```python
from build123d import *

# Parameters (mm, degrees)
SKETCH_1_R      = 10
EXTRUDE_1_DEPTH = 20
SKETCH_3_R      = 9
EXTRUDE_3_DEPTH = 20


with BuildPart() as part:
    # 草圖1 → 填料-伸長1 (new body)
    with BuildSketch(Plane(origin=(0, 0, 0), x_dir=(1, 0, 0), z_dir=(0, 1, 0))):
        with BuildLine():
            Line((0, 0), (150, 0))
            Line((150, 0), (150, -48.937372985))
            ThreePointArc((150, -48.937372985), (142.306045532, -66.979013377), (123.959936956, -73.915728993))
            Line((123.959936956, -73.915728993), (14.009507708, -39.398116187))
            ThreePointArc((14.009507708, -39.398116187), (3.878432988, -32.15252135), (0, -20.316344726))
            Line((0, -20.316344726), (0, 0))
        make_face()
        with Locations(Location((20, -19.398116187, 0), (0, 0, 270))):
            Circle(SKETCH_1_R, mode=Mode.SUBTRACT)
        with Locations(Location((125, -48.915728993, 0), (0, 0, 270))):
            Circle(SKETCH_1_R, mode=Mode.SUBTRACT)
    extrude(amount=EXTRUDE_1_DEPTH)

    # 草圖3 → 填料-伸長3 (add)
    with BuildSketch(Plane(origin=(0, 0, 0), x_dir=(-1, 0, 0), z_dir=(0, 0, -1))):
        with BuildLine():
            Line((-150, 20), (-150, 50.956093838))
            ThreePointArc((-150, 50.956093838), (-147.247819565, 58.603173888), (-140.253694451, 62.742563256))
            Line((-140.253694451, 62.742563256), (-79.695196774, 74.321972269))
            ThreePointArc((-79.695196774, 74.321972269), (-59.068583229, 69.033118411), (-50, 49.76682765))
            Line((-50, 49.76682765), (-50, 20))
            Line((-50, 20), (-150, 20))
        make_face()
        with Locations((-75, 49.76682765)):
            Circle(SKETCH_3_R, mode=Mode.SUBTRACT)
    extrude(amount=-EXTRUDE_3_DEPTH)


solid = part.part
```
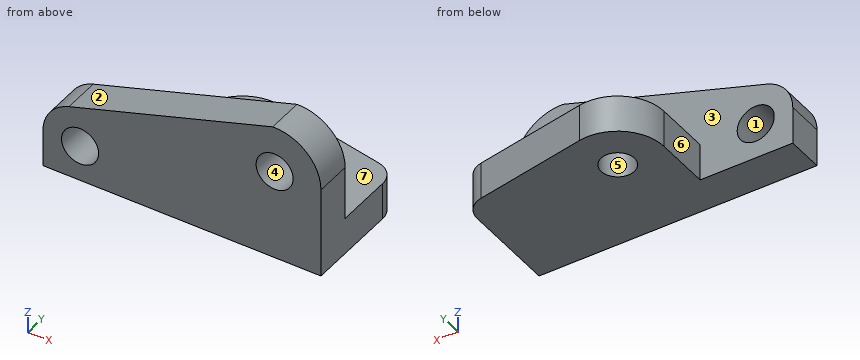
The model under review builds one solid part; all positions refer to its coordinate system, in mm. Face numbers are marked on the shaded views. A direction names the side the tool comes from. Round coordinates to 2 decimals unless told otherwise and drop trailing zeros. Write each loop counter-clockwise with the first axis right and the second up, starting at its lowest first coordinate (ties: lowest second). Pieces come first, ordered by that corner, then holes. Notation, with made-up numbers: M -25.5,-16.75 L 18.5,-16.75 A30 ccw 18.5,16.25 Z; hole C -3,57.5 d7. An arc over 180 degrees is marked long. Use CSV: the item, a comma, the result in double quotes. Start each with the question number.
(1) We need section C-C, the plane z = 54. State the section outline as (x, y) points, then the cut area to 3 significant figures.
(2) Clearance check with flat-ended pins moving along their axes: P1, Ø5, axis at x = 110.5, y = 51.5, coming from the +Z side; P2, Ø8, axis at y = 54, z = 13.5, coming from the +X side; P3, Ø1, axis at x = 117, y = 15.5, coming from the +Z side; P4, Ø6, axis at x = 64.5, z = 13, coming from the +Y side. State where each tip first meets the part, or that it passes through.
(3) Tool access review of the marked faces 5, 6 and 7: name each direction out of +Z, -Z, +X, -X, +Y, -Y from which nothing blocks a thin tool from reaching the whole face with its end or side.
(4) We need section A-A, the plane y = 18. State the section outline as (x, z) points.
(5) We need section D-D, the plane z = 5. State the section outline as (x, y) points, then the cut area to 3 significant figures.
(6) The part is to be moulded in two halves that separate along Z. For the marked faces 1, 2, 3 and 4, say which applies: +Z half, -Z half, draft (parallel to the pull), parting line (faces both ways), or undercut.
(7) For line 1 along Y through (x, z) = (75, 15.25); line 2 along Z through (x, y) = (95, 60); line 3 along X through (y, z) = (15.5, 18), list the stretches that pass through material, from the lowest coordinate up.
(8) We need section B-B, the plane x = 70.5. State the section outline as (y, z) points.
Findings:
1,outline,"M 60.52,0 L 116.39,0 L 116.39,20 L 60.52,20 Z; M 133.61,0 L 149.48,0 L 149.48,20 L 133.61,20 Z"
1,area,"1,430 mm^2"
2,P1,"z = 20"
2,P2,"x = 150"
2,P3,"z = 71.89"
2,P4,"y = 73.62"
3,face 5,"+Z, -Z"
3,face 6,"+Z, -Z, -X, +Y"
3,face 7,"+Z, +X, -X, +Y"
4,outline,"M 0,0 L 150,0 L 150,48.94 A25 ccw 123.96,73.92 L 14.01,39.4 A20 ccw 0,20.32 Z; hole C 20,19.4 d20; hole C 125,48.92 d20"
5,outline,"M 0,0 L 150,0 L 150,50.96 A12 ccw 140.25,62.74 L 79.7,74.32 A25 ccw 50,49.77 L 50,20 L 0,20 Z; hole C 75,49.77 d18"
5,area,"7,560 mm^2"
6,face 1,"undercut"
6,face 2,"+Z half"
6,face 3,"draft"
6,face 4,"undercut"
7,line 1,"0 to 40.77, 58.77 to 74.77"
7,line 2,"0 to 20"
7,line 3,"0 to 10.1, 29.9 to 150"
8,outline,"M 0,0 L 41.97,0 L 41.97,20 L 20,20 L 20,57.13 L 0,57.13 Z; M 57.56,0 L 74.36,0 L 74.36,20 L 57.56,20 Z"
